Design review of the part built by this model. Coordinates are the model's own, in mm. A direction names the side the tool comes from. Coordinates: 2 decimals unless noted, no trailing zeros. Order: outer loops, then holes, each group sorted by start corner. A loop starts at its lowest first (then second) coordinate and runs counter-clockwise, first axis right, second up. Notation, with made-up numbers: M -13,85 L 46,85 A23 cw 46,121 Z; hole C 14.5,87 d4. An arc over 180 degrees is marked long. Answer in a Markdown table with one row per item.
from build123d import *

# Parameters (mm, degrees)
F1_DEPTH = 6.35
F3_R     = 2.54
F4_DEPTH = 6.35
F5_DEPTH = 6.35
F6_DEPTH = 6.35
F7_DEPTH = 19.05


with BuildPart() as f1:
    # F0 (on Top) → F1 (new body)
    with BuildSketch(Plane.XY):
        Polygon((31.1166602765, 114.2971263717), (-38.7333397235, 114.2971263717), (-39.0034913485, 101.6), (-10.4284913485, 101.6), (-10.4284913485, -12.7), (2.5416602765, -12.7), (2.5416602765, 101.6), (31.1166602765, 101.6), align=None)
    extrude(amount=F1_DEPTH)

    # F3
    f3_edges = [f1.edges().sort_by_distance(p)[0] for p in [
        (-24.715991, 101.6, 6.35),
        (-38.868416, 107.948563, 6.35),
        (-3.80834, 114.297126, 6.35),
        (16.82916, 101.6, 6.35),
        (31.11666, 107.948563, 6.35),
        (2.54166, 44.45, 6.35),
        (-10.428491, 44.45, 6.35),
        (-3.943416, -12.7, 6.35),
        (-24.715991, 101.6, 0),
        (-38.868416, 107.948563, 0),
        (-3.80834, 114.297126, 0),
        (16.82916, 101.6, 0),
        (31.11666, 107.948563, 0),
        (2.54166, 44.45, 0),
        (-10.428491, 44.45, 0),
        (-3.943416, -12.7, 0),
    ]]
    fillet(f3_edges, radius=F3_R)

    # F2 (on face) → F4 (cut)
    with BuildSketch(Plane.XY.offset(6.35)):
        with BuildLine():
            Line((-27.6843397235, 108.3281263717), (-29.2718397235, 108.3281263717))
            Line((-29.2718397235, 108.3281263717), (-30.8593397235, 108.3281263717))
            ThreePointArc((-30.8593397235, 108.3281263717), (-29.2718397235, 106.7406263717), (-27.6843397235, 108.3281263717))
        make_face()
        with BuildLine():
            Line((-30.8593397235, 108.3281263717), (-29.2718397235, 108.3281263717))
            Line((-29.2718397235, 108.3281263717), (-27.6843397235, 108.3281263717))
            ThreePointArc((-27.6843397235, 108.3281263717), (-29.2718397235, 109.9156263717), (-30.8593397235, 108.3281263717))
        make_face()
    extrude(amount=-F4_DEPTH, mode=Mode.SUBTRACT)

    # F2 (on face) → F5 (cut)
    with BuildSketch(Plane.XY.offset(6.35)):
        with BuildLine():
            ThreePointArc((21.7121915103, 109.904923364), (20.4726967133, 109.5139395597), (19.9406602765, 108.3281263717))
            Line((19.9406602765, 108.3281263717), (21.5281602765, 108.3281263717))
            Line((21.5281602765, 108.3281263717), (21.7121915103, 108.3281263717))
            Line((21.7121915103, 108.3281263717), (21.7121915103, 109.904923364))
        make_face()
        with BuildLine():
            ThreePointArc((23.1156602765, 108.3281263717), (22.7139734645, 109.3835899349), (21.7121915103, 109.904923364))
            Line((21.7121915103, 109.904923364), (21.7121915103, 108.3281263717))
            Line((21.7121915103, 108.3281263717), (23.1156602765, 108.3281263717))
        make_face()
        with BuildLine():
            Line((21.7121915103, 108.3281263717), (21.7121915103, 106.7513293794))
            ThreePointArc((21.7121915103, 106.7513293794), (22.7139734645, 107.2726628086), (23.1156602765, 108.3281263717))
            Line((23.1156602765, 108.3281263717), (21.7121915103, 108.3281263717))
        make_face()
        with BuildLine():
            Line((21.5281602765, 108.3281263717), (19.9406602765, 108.3281263717))
            ThreePointArc((19.9406602765, 108.3281263717), (20.4726967133, 107.1423131837), (21.7121915103, 106.7513293794))
            Line((21.7121915103, 106.7513293794), (21.7121915103, 108.3281263717))
            Line((21.7121915103, 108.3281263717), (21.5281602765, 108.3281263717))
        make_face()
    extrude(amount=-F5_DEPTH, mode=Mode.SUBTRACT)

    # F2 (on face) → F6 (cut)
    with BuildSketch(Plane.XY.offset(6.35)):
        with BuildLine():
            Line((-3.8718397235, 65.912123364), (-3.8718397235, 67.499623364))
            ThreePointArc((-3.8718397235, 67.499623364), (-5.4593397235, 65.912123364), (-3.8718397235, 64.324623364))
            Line((-3.8718397235, 64.324623364), (-3.8718397235, 65.912123364))
        make_face()
        with BuildLine():
            ThreePointArc((-2.2843397235, 65.912123364), (-2.7493077084, 67.0346553792), (-3.8718397235, 67.499623364))
            Line((-3.8718397235, 67.499623364), (-3.8718397235, 65.912123364))
            Line((-3.8718397235, 65.912123364), (-2.2843397235, 65.912123364))
        make_face()
        with BuildLine():
            ThreePointArc((-3.8718397235, 64.324623364), (-2.7493077084, 64.7895913489), (-2.2843397235, 65.912123364))
            Line((-2.2843397235, 65.912123364), (-3.8718397235, 65.912123364))
            Line((-3.8718397235, 65.912123364), (-3.8718397235, 64.324623364))
        make_face()
    extrude(amount=-F6_DEPTH, mode=Mode.SUBTRACT)

    # F2 (on face) → F7 (join)
    with BuildSketch(Plane.XY.offset(6.35)):
        with BuildLine():
            Line((-3.8718397235, -3.937876636), (-3.8718397235, -1.397876636))
            ThreePointArc((-3.8718397235, -1.397876636), (-6.4118397235, -3.937876636), (-3.8718397235, -6.477876636))
            Line((-3.8718397235, -6.477876636), (-3.8718397235, -3.937876636))
        make_face()
        with BuildLine():
            ThreePointArc((-1.3318397235, -3.937876636), (-2.0757884993, -2.1418254117), (-3.8718397235, -1.397876636))
            Line((-3.8718397235, -1.397876636), (-3.8718397235, -3.937876636))
            Line((-3.8718397235, -3.937876636), (-1.3318397235, -3.937876636))
        make_face()
        with BuildLine():
            Line((-1.3318397235, -3.937876636), (-3.8718397235, -3.937876636))
            Line((-3.8718397235, -3.937876636), (-3.8718397235, -6.477876636))
            ThreePointArc((-3.8718397235, -6.477876636), (-2.0757884993, -5.7339278602), (-1.3318397235, -3.937876636))
        make_face()
    extrude(amount=F7_DEPTH)


solid = f1.part
(1) For faces 1 (the cylindrical face through (-9.7, 44.9, 0.76)), 2 (the cylindrical face through (-9.7, 44.9, 5.59)), 3 (the cylindrical face through (15.777, 102.324, 5.586)), 4 (the cylindrical face through (15.777, 102.324, 0.764)), list the 3-axis set-ups (+Z, -Z, +X, -X, +Y, -Y) from which the entire face can be reached by the end or side of a thin tool; tool diameter is ignored.
Return value:
| item | result |
|---|---|
| face 1 | -Z, -X, -Y |
| face 2 | +Z, -X, -Y |
| face 3 | +Z, +X, -Y |
| face 4 | -Z, +X, -Y |
(2) For line 1 along X through (y, z) = (48, 2.25); line 2 along Z through (x, y) = (-5, 40); line 3 along Z through (x, y) = (2, 28), list the stretches that pass through material, from the lowest coordinate up. Write a range as from..to.
Return value:
| item | result |
|---|---|
| line 1 | x = -10.41..2.53 |
| line 2 | z = 0..6.35 |
| line 3 | z = 0.97..5.38 |
(3) Add section C-C, the plane x = -29. Give the boundary of the cut face in (y, z), and give its area (3 significant figures).
Return value:
| item | result |
|---|---|
| outline | M 101.6,2.54 A2.54 ccw 104.14,0 L 106.76,0 L 106.76,6.35 L 104.14,6.35 A2.54 ccw 101.6,3.81 Z; M 109.89,0 L 111.76,0 A2.54 ccw 114.3,2.54 L 114.3,3.81 A2.54 ccw 111.76,6.35 L 109.89,6.35 Z |
| area | 55.2 mm2 |
(4) Insertion check: pin 1 Ø0.6 at (x, z) = (-23.5, 3) entering from -Y; pin 2 Ø3 at (x, y) = (-10, 99.5) entering from -Z; pin 3 Ø12 at (x, z) = (14, 11) entering from -Y. Each pin has a flat end and moves straight along its axis. Give the tip position at first contact, or say it passes through.
Return value:
| item | result |
|---|---|
| pin 1 | stops at y = 101.6 |
| pin 2 | stops at z = 0.07 |
| pin 3 | stops at y = 101.9 |
(5) Add section B-B, the plane y = 56. Give the boundary of the cut face in (x, z).
Return value:
| item | result |
|---|---|
| outline | M -10.43,2.54 A2.54 ccw -7.89,0 L 0,0 A2.54 ccw 2.54,2.54 L 2.54,3.81 A2.54 ccw 0,6.35 L -7.89,6.35 A2.54 ccw -10.43,3.81 Z |
(6) Draft analysis for pull direction X (two halves, no side actions). For faces 5 (the cylindrical face through (-29.62, 106.78, 3.22)), 6 (the cylindrical face through (-38.146, 107.844, 0.764)), 7 (the cylindrical face through (-4.3, 113.57, 5.59)), 8 (the cylindrical face through (30.39, 108.04, 5.59)), state which applies: pulls with the +X half, pulls with the -X half, needs draft (parallel to the pull), parting line crosses it, or undercut.
Return value:
| item | result |
|---|---|
| face 5 | undercut |
| face 6 | pulls with the -X half |
| face 7 | needs draft |
| face 8 | pulls with the +X half |
(7) Add section D-D, the plane z = 14. Give the boundary of the cut face in (x, y), and give its area (3 significant figures).
Return value:
| item | result |
|---|---|
| outline | C -3.87,-3.94 d5.08 |
| area | 20.3 mm2 |
(8) Add section A-A, the plane x = 15. Give the boundary of the cut face in (y, z).
Return value:
| item | result |
|---|---|
| outline | M 101.6,2.54 A2.54 ccw 104.14,0 L 111.76,0 A2.54 ccw 114.3,2.54 L 114.3,3.81 A2.54 ccw 111.76,6.35 L 104.14,6.35 A2.54 ccw 101.6,3.81 Z |
